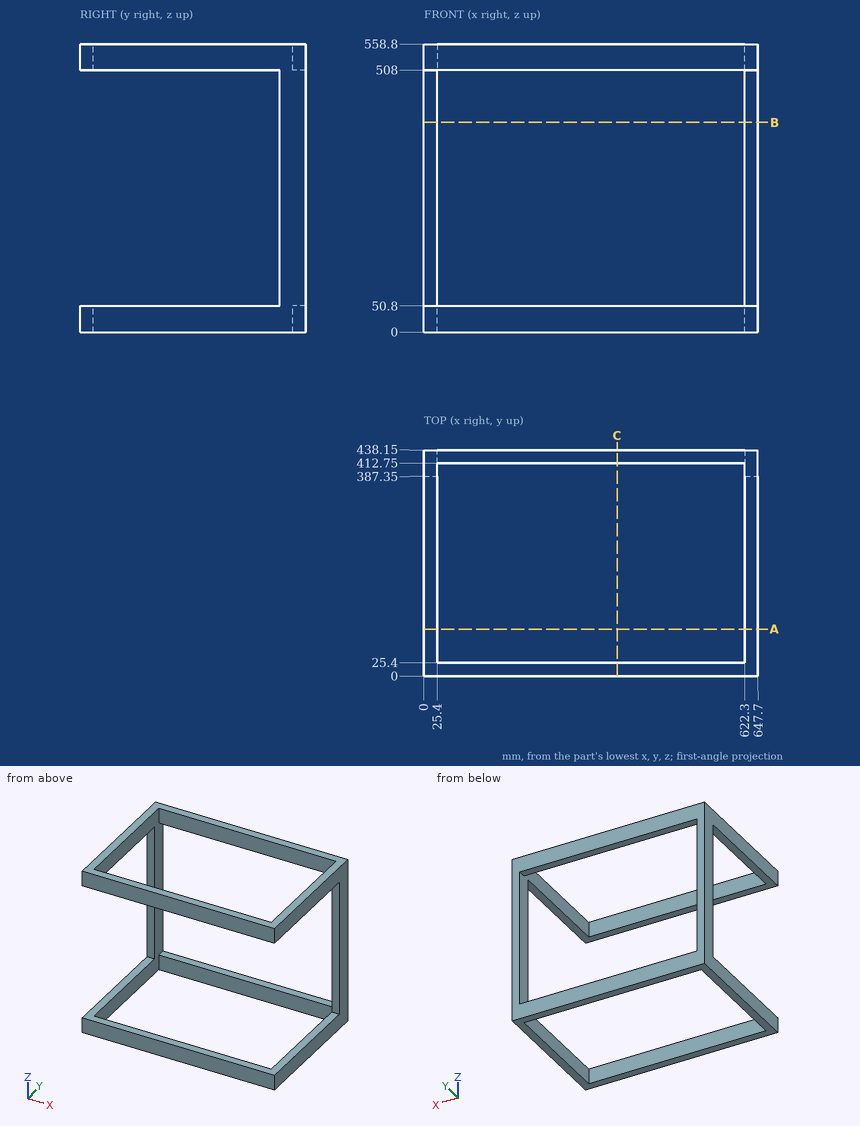
Check sheet for the drawn part. Datum: minimum x, y, z corner. Units: mm. Round coordinates to 2 decimals unless told otherwise and drop trailing zeros. Order: outer loops, then holes, each group sorted by start corner. A loop starts at its lowest first (then second) coordinate and runs counter-clockwise, first axis right, second up. Notation, with made-up numbers: (65, 70) - (76, 70) arc R23 cw to (76, 103) - close; hole circle Ø1 at (-26, -2.75). An arc over 180 degrees is marked (long way). Use a Markdown table: item, result. Add a question column.
(1) Sectioned sample at C-C, the plane x = 374.5. Enter the section's corners in (y, z), and give its area (3 significant figures).
(2) Sectioned sample at A-A, the plane y = 91. Enter the section's corners in (x, z).
(3) Depth check by flat-ended pin: pin 1 (7.5 mm diameter, centred on x = 632, z = 259, fed in from -Y). Enter the tip coordinate at first touch or a pass-through.
(4) Material ranges on line 1 along X through (y, z) = (392, 404); line 2 along Z through (x, y) = (522.5, 420.5); line 3 along Y through (x, z) = (68.5, 522), recorded low to high. Write a range as [from, to].
(5) Sectioned sample at B-B, the plane z = 407. Enter the section's corners in (x, y).
Answers below:
| question | item | result |
|---|---|---|
| 1 | outline | (0, 0) - (25.4, 0) - (25.4, 50.8) - (0, 50.8) - close; (0, 508) - (25.4, 508) - (25.4, 558.8) - (0, 558.8) - close; (412.75, 0) - (438.15, 0) - (438.15, 50.8) - (412.75, 50.8) - close; (412.75, 508) - (438.15, 508) - (438.15, 558.8) - (412.75, 558.8) - close |
| 1 | area | 5,160 mm² |
| 2 | outline | (0, 0) - (25.4, 0) - (25.4, 50.8) - (0, 50.8) - close; (0, 508) - (25.4, 508) - (25.4, 558.8) - (0, 558.8) - close; (622.3, 0) - (647.7, 0) - (647.7, 50.8) - (622.3, 50.8) - close; (622.3, 508) - (647.7, 508) - (647.7, 558.8) - (622.3, 558.8) - close |
| 3 | pin 1 | y = 387.35 |
| 4 | line 1 | [0, 25.4], [622.3, 647.7] |
| 4 | line 2 | [0, 50.8], [508, 558.8] |
| 4 | line 3 | [0, 25.4], [412.75, 438.15] |
| 5 | outline | (0, 387.35) - (25.4, 387.35) - (25.4, 438.15) - (0, 438.15) - close; (622.3, 387.35) - (647.7, 387.35) - (647.7, 438.15) - (622.3, 438.15) - close |
